Input: part model. Units: mm. Frame: model coordinates. A direction names the side the tool comes from. Coordinates: 2 decimals unless noted, no trailing zeros. Loops run counter-clockwise (first coordinate to the right, second up) from the corner with the lowest first, then second, coordinate; pieces in that order, holes last. Notation, with made-up numbers: (29, 82) -> (87, 82) arc R17 cw to (87, 104) -> close; hole circle Ø11 at (66, 22.25). An arc over 180 degrees is marked (long way). Answer as a JSON object with one key per item and string values.
Autodesk Inventor part; units mm, degrees
ref_plane "YZ Plane" through (0, 0, 0) normal (1, 0, 0) x (0, 1, 0)
ref_plane "XZ Plane" through (0, 0, 0) normal (0, 1, 0) x (-1, 0, 0)
ref_plane "XY Plane" through (0, 0, 0) normal (0, 0, 1) x (1, 0, 0)
sketch "Sketch1" plane through (0, 0, 0) normal (1, 0, 0) x (0, 1, 0)
  line L0 (12.5, 55) -> (-12.5, 55)
  line L1 (-12.5, 55) -> (-12.5, -55)
  line L2 (-12.5, -55) -> (12.5, -55)
  line L3 (12.5, -55) -> (12.5, 55)
  arc A0 (12.5, 55) -> (-12.5, 55) centre (0, 55) ccw
  arc A1 (-12.5, -55) -> (12.5, -55) centre (0, -55) ccw
  circle A2 centre (0, 55) radius 1.65
  circle A3 centre (0, 55) radius 3.75
  circle A4 centre (0, 55) radius 8.25
  line L4 (4, 55) -> (-4, 55)
  line L5 (-4, 55) -> (-4, 27.25)
  line L6 (-4, 27.25) -> (4, 27.25)
  line L7 (4, 27.25) -> (4, 55)
  circle A5 centre (0, 31) radius 1.65
  circle A6 centre (0, 36) radius 1.65
  line L8 (1.65, 36) -> (1.65, 31)
  line L9 (-1.65, 36) -> (-1.65, 31)
  line L10 (12.5, 0) -> (-12.5, 0) construction
  circle A7 centre (0, -55) radius 1.65
  circle A8 centre (0, -55) radius 3.75
  circle A9 centre (0, -55) radius 8.25
  line L11 (-4, -55) -> (-4, -27.25)
  line L12 (-4, -27.25) -> (4, -27.25)
  line L13 (4, -27.25) -> (4, -55)
  circle A10 centre (0, -31) radius 1.65
  circle A11 centre (0, -36) radius 1.65
  line L14 (1.65, -36) -> (1.65, -31)
  line L15 (-1.65, -36) -> (-1.65, -31)
  line L16 (4.5, 25) -> (-4.5, 25)
  line L17 (-4.5, 25) -> (-4.5, -25)
  line L18 (-4.5, -25) -> (4.5, -25)
  line L19 (4.5, -25) -> (4.5, 25)
  line L20 (4.5, 25) -> (-4.5, -25) construction
  line L21 (-4.5, 25) -> (4.5, -25) construction
  arc A12 (-4.5, 25) -> (4.5, 25) centre (0, 33.9303) ccw
  arc A13 (4.5, -25) -> (-4.5, -25) centre (0, -33.9303) ccw
  point P0 (0, 0)
  point P1 (0, 55)
  point P2 (-4, -47.7846)
  point P3 (4, -47.7846)
  point P4 (4, 47.7846)
  point P5 (-4, 47.7846)
  point P6 (0, 0)
  point P7 (3.75, 55)
  point P8 (-3.75, 55)
  dimension "d0" = 110
  dimension "d1" = 55
  dimension "d2" = 12.5
  dimension "d3" = 25
  dimension "d4" = 3.3
  dimension "d5" = 7.5
  dimension "d6" = 16.5
  dimension "d7" = 8
  dimension "d8" = 4
  dimension "d10" = 36
  dimension "d11" = 3.3
  dimension "d12" = 24
  dimension "d13" = 4
  dimension "d14" = 3.3
  dimension "d15" = 5
  dimension "d16" = 4
  dimension "d34" = 50
  dimension "d35" = 8
  dimension "d36" = 8
  dimension "d37" = 10
  dimension "d38" = 10
extrude "Extrusion1" add sketch "Sketch1" along normal blind 4.5 contours L3 L2 A9 L13 L12 L11 L1 L0 A4 L5 L6 L7 | L0 A4 A0 | A1 L2 A9 | A12 L16 | L18 A13
extrude "Extrusion2" add sketch "Sketch1" against normal blind 1.5 contours L3 L2 A9 L13 L12 L11 L1 L0 A4 L5 L6 L7 | L0 A4 A0 | A4 L7 L0 | L0 A3 A4 | A1 L2 A9 | L7 A4 L5 L0 A3 | L0 L5 A4 | L7 L6 L5 A4 | A9 L2 A8 | L2 L13 A9 | A3 L0 A2 | L0 A2 A3 | L2 A8 L11 A9 L13 | A9 L11 L12 L13 | A9 L11 L2 | A8 L2 A7 | L2 A7 A8 | A12 L16 | L18 A13
extrude "Extrusion3" add sketch "Sketch1" along normal blind 1 contours A3 L0 A2 | L0 A2 A3 | A8 L2 A7 | L2 A7 A8
fillet "Fillet1" radius 4 4 edges at (2.25, -4, 27.25) (2.25, 4, 27.25) (2.25, -4, -27.25) (2.25, 4, -27.25)
fillet "Fillet2" radius 8 4 edges at (2.25, -4, -47.7846) (2.25, 4, -47.7846) (2.25, -4, 47.7846) (2.25, 4, 47.7846)
fillet "Fillet3" radius 2 8 edges at (4.5, 0, 67.5) (4.5, -12.5, 0) (4.5, 0, -67.5) (4.5, 12.5, 0) (-1.5, 0, -67.5) (-1.5, -12.5, 0) (-1.5, 0, 67.5) (-1.5, 12.5, 0)
equation "\"d0\" = FEMUR_X"
equation "\"d3\" = FEMUR_WIDTH"
equation "\"d4\" = HornScrewDiameter"
equation "\"d5\" = HornCentreDiameter"
equation "\"d6\" = HornDiameter"
equation "\"d7\" = HornWidth"
equation "\"d8\" = 0.5 * HornWidth"
equation "\"d10\" = HornLength"
equation "\"d11\" = HornScrewDiameter"
equation "\"d13\" = 0.5 * HornWidth"
equation "\"d14\" = HornScrewDiameter"
equation "\"d15\" = HornScrewLen"
equation "\"d16\" = 0.5 * HornWidth"
equation "\"d17\" = FEMUR_HEIGHT - HORN_HEIGHT"
equation "\"d19\" = HORN_HEIGHT"
equation "\"d21\" = HornCentreHeight"
equation "\"d23\" = 0.5 * HornWidth"
equation "\"d24\" = HornFillet"
equation "\"d25\" = PART_FILLET"
properties part number "FemurHornSide"
1. Access query for faces 4 (the face through (1, -4.5, 0)), 5 (the face through (2.218, 0.267, -63.246)). Directions: +Z, -Z, +X, -X, +Y, -Y. A direction counts if a zero-diameter tool reaches every point of the face in a straight line with its end or side. Return the directions, or none.
Reply:
{"face 4": "+X, -X", "face 5": "+X"}
2. Section query A-A (z = -11). Return loops of the section in (x, y).
Reply:
{"outline": "(-1.5, -10.5) arc R2 ccw to (0.5, -12.5) -> (2.5, -12.5) arc R2 ccw to (4.5, -10.5) -> (4.5, -4.5) -> (-1.5, -4.5) -> close; (-1.5, 4.5) -> (4.5, 4.5) -> (4.5, 10.5) arc R2 ccw to (2.5, 12.5) -> (0.5, 12.5) arc R2 ccw to (-1.5, 10.5) -> close"}
3. Pin query (flat end, axial travel): P1, Ø6, axis at y = 0.5, z = 55.5, coming from the +X side; P2, Ø1.6, axis at x = -1, z = 34.5, coming from the -Y side; P3, Ø3, axis at x = 0.5, y = 3.5, coming from the +Z side. Return the tip coordinate at first contact, or that it passes through.
Reply:
{"P1": "stops at x = 1", "P2": "stops at y = -12.37", "P3": "stops at z = 67.34"}
4. Line query: line 1 along Z through (x, y) = (3.5, 2); line 2 along Y through (x, z) = (1.1, 55); line 3 along Y through (x, z) = (2.5, 36). Output: solid intervals per line, ascending.
Reply:
{"line 1": "z = -67.07 to -63, -27.79 to -24.13, 24.13 to 27.79, 63 to 67.07", "line 2": "y = -12.5 to -8.25, 8.25 to 12.5", "line 3": "y = -12.5 to -4, 4 to 12.5"}
5. Mould query, pull axis Z, two halves, no side actions, for faces 1 (the face through (2.282, -4.527, 46.897)), 2 (the face through (1.486, -0.275, 67.497)), 3 (the face through (4.5, -5, 1)). Classes: pulls with the +Z half, pulls with the -Z half, needs draft (parallel to the pull), parting line crosses it, or undercut.
Reply:
{"face 1": "undercut", "face 2": "pulls with the +Z half", "face 3": "needs draft"}
